Autodesk Inventor part; units mm, degrees
ref_plane "YZ Plane" through (0, 0, 0) normal (1, 0, 0) x (0, 1, 0)
ref_plane "XZ Plane" through (0, 0, 0) normal (0, 1, 0) x (-1, 0, 0)
ref_plane "XY Plane" through (0, 0, 0) normal (0, 0, 1) x (1, 0, 0)
sketch "Sketch1" plane through (0, 0, 0) normal (0, 1, 0) x (-1, 0, 0)
  circle A0 centre (0, 0) radius 13
  line L0 (-14.9666, 24.75) -> (-24.75, 14.9666)
  line L1 (-24.75, 14.9666) -> (-24.75, -14.9666) construction
  line L2 (-24.75, -14.9666) -> (-14.9666, -24.75)
  line L3 (-14.9666, -24.75) -> (14.9666, -24.75) construction
  line L4 (14.9666, -24.75) -> (24.75, -14.9666)
  line L5 (24.75, -14.9666) -> (24.75, 14.9666) construction
  line L6 (24.75, 14.9666) -> (14.9666, 24.75)
  line L7 (14.9666, 24.75) -> (-14.9666, 24.75) construction
  arc A1 (-24.75, -14.9666) -> (-24.75, 14.9666) centre (-50.75, 0) ccw
  arc A2 (-14.9666, 24.75) -> (14.9666, 24.75) centre (0, 50.75) ccw
  arc A3 (24.75, 14.9666) -> (24.75, -14.9666) centre (50.75, 0) ccw
  arc A4 (14.9666, -24.75) -> (-14.9666, -24.75) centre (0, -50.75) ccw
  circle A5 centre (-15, 15) radius 4
  circle A6 centre (15, 15) radius 4
  circle A7 centre (15, -15) radius 4
  circle A8 centre (-15, -15) radius 4
  point P0 (-24.75, 0)
  point P1 (24.75, 0)
  point P2 (0, 24.75)
  point P3 (0, -24.75)
  point P4 (0, 20.75)
  dimension "d0" = 26
  dimension "d1" = 49.5
  dimension "d2" = 30
  dimension "d3" = 4
  dimension "d4" = 30
  dimension "d5" = 30
  dimension "d6" = 15
  dimension "d7" = 15
  dimension "d8" = 8
extrude "Extrusion1" add sketch "Sketch1" along normal blind 7
fillet "Fillet1" radius 3 8 edges at (24.75, 3.5, 14.9666) (14.9666, 3.5, 24.75) (-14.9666, 3.5, 24.75) (-24.75, 3.5, 14.9666) (-24.75, 3.5, -14.9666) (-14.9666, 3.5, -24.75) (14.9666, 3.5, -24.75) (24.75, 3.5, -14.9666)
equation "\"d5\" = d4"
properties part number "WobbleX WS12" material "Aluminum 6061"
Verification items for the finished model (mm, model axes). Round coordinates to 2 decimals unless told otherwise and drop trailing zeros. Write each loop counter-clockwise with the first axis right and the second up, starting at its lowest first coordinate (ties: lowest second). Pieces come first, ordered by that corner, then holes.
1. Section check D-D on z = -15. Enter the section's corners in (x, y), plus the area to 3 significant figures.
2. Scan lines: L1, parallel to Z at x = 15, y = 5.5; L2, parallel to Z at x = -14, y = 3.5; L3, parallel to X at y = 6.25, z = -18. Record each from-to range of solid material in increasing order.
3. Draft check along Z on faces 1 (the cylindrical face through (14.935, 3.549, -24.017)), 2 (the cylindrical face through (-0.19, 3.45, 20.75)), 3 (the cylindrical face through (17.95, 3.45, -17.7)). Enter one of: +Z half, -Z half, draft (parallel to the pull), parting line (faces both ways), or undercut.
4. Gauge pin test, flat ends, axial feed: P1, Ø1.5, axis at y = 6.5, z = -7.5, coming from the +X side; P2, Ø2, axis at y = 5, z = -18.5, coming from the -X side; P3, Ø10.5, axis at x = -15, z = -15, coming from the -Y side; P4, Ø1.5, axis at x = 8, y = 2, coming from the -Z side. Record the tip position at first contact, or that the pin passes through.
5. Section check A-A on x = 0. Enter the section's corners in (y, z).
6. Section check B-B on z = 0. Enter the section's corners in (x, y).
7. Section check C-C on y = 3. Enter the section's corners in (x, z).
Answer:
1. outline: (-24, 0) - (-19, 0) - (-19, 7) - (-24, 7) - close; (-11, 0) - (11, 0) - (11, 7) - (-11, 7) - close; (19, 0) - (24, 0) - (24, 7) - (19, 7) - close
1. area: 224 mm2
2. L1: z = -24 to -19, -11 to 11, 19 to 24
2. L2: z = -24.03 to -18.87, -11.13 to 11.13, 18.87 to 24.03
2. L3: x = -21.72 to -17.65, -12.35 to 12.35, 17.65 to 21.72
3. face 1: -Z half
3. face 2: +Z half
3. face 3: undercut
4. P1: stops at x = 21.91
4. P2: stops at x = -22.22
4. P3: stops at y = 0
4. P4: stops at z = -22.05
5. outline: (0, -20.75) - (7, -20.75) - (7, -13) - (0, -13) - close; (0, 13) - (7, 13) - (7, 20.75) - (0, 20.75) - close
6. outline: (-20.75, 0) - (-13, 0) - (-13, 7) - (-20.75, 7) - close; (13, 0) - (20.75, 0) - (20.75, 7) - (13, 7) - close
7. outline: (-23.76, -13.1) arc R3 ccw to (-23.18, -16.53) - (-16.53, -23.18) arc R3 ccw to (-13.1, -23.76) arc R30 cw to (13.1, -23.76) arc R3 ccw to (16.53, -23.18) - (23.18, -16.53) arc R3 ccw to (23.76, -13.1) arc R30 cw to (23.76, 13.1) arc R3 ccw to (23.18, 16.53) - (16.53, 23.18) arc R3 ccw to (13.1, 23.76) arc R30 cw to (-13.1, 23.76) arc R3 ccw to (-16.53, 23.18) - (-23.18, 16.53) arc R3 ccw to (-23.76, 13.1) arc R30 cw to start; hole circle Ø8 at (-15, -15); hole circle Ø8 at (-15, 15); hole circle Ø26 at (0, 0); hole circle Ø8 at (15, -15); hole circle Ø8 at (15, 15)
